from build123d import *

# Parameters (mm, degrees)
F1_R     = 13.2
F2_DEPTH = 7


with BuildPart() as f2:
    # F1 (on Top) → F2 (new body)
    with BuildSketch(Plane.XY):
        with BuildLine():
            ThreePointArc((10.821909, 27.530935), (10.756845, 27.278632), (10.694101, 27.025743))
            ThreePointArc((10.694101, 27.025743), (10.76097, 27.277589), (10.821909, 27.530935))
        make_face()
        with BuildLine():
            ThreePointArc((23.829551, -4.11045), (12.121504, 9.289095), (10.694101, 27.025743))
            ThreePointArc((10.694101, 27.025743), (10.756845, 27.278632), (10.821909, 27.530935))
            ThreePointArc((10.821909, 27.530935), (0, 41.1), (-10.821909, 27.530935))
            ThreePointArc((-10.821909, 27.530935), (-10.756845, 27.278632), (-10.694101, 27.025743))
            ThreePointArc((-10.694101, 27.025743), (-12.121504, 9.289095), (-23.829551, -4.11045))
            ThreePointArc((-23.829551, -4.11045), (-35.415268, -20.848085), (-15.271056, -17.917565))
            ThreePointArc((-15.271056, -17.917565), (0.00942, -15.335501), (15.28268, -17.959904))
            ThreePointArc((15.28268, -17.959904), (35.426816, -20.829414), (23.829551, -4.11045))
        make_face()
        Circle(F1_R, mode=Mode.SUBTRACT)
        with BuildLine():
            ThreePointArc((-10.694101, 27.025743), (-10.756845, 27.278632), (-10.821909, 27.530935))
            ThreePointArc((-10.821909, 27.530935), (-10.76097, 27.277589), (-10.694101, 27.025743))
        make_face()
    extrude(amount=F2_DEPTH)


solid = f2.part
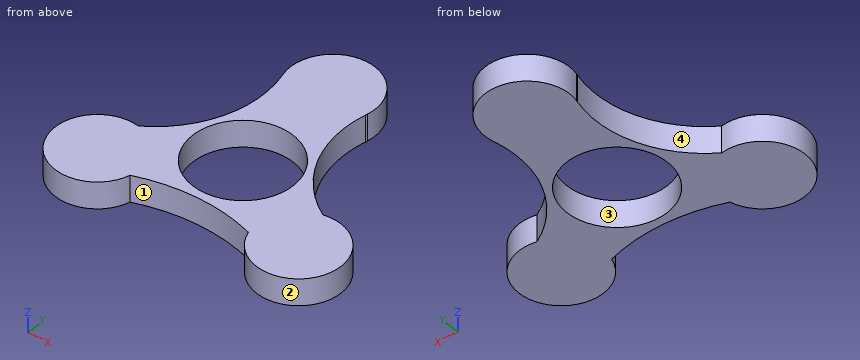
Part model, mm, in its own coordinate system. Face numbers are marked on the shaded views. Coordinates: 2 decimals unless noted, no trailing zeros. Order: outer loops, then holes, each group sorted by start corner. A loop starts at its lowest first (then second) coordinate and runs counter-clockwise, first axis right, second up.
(1) Slice it at B-B, the plane z = 2. Write the cut outline in (x, y), and give its area (3 significant figures).
Check sheet entries:
outline: (-23.83, -4.11) arc R11.1 ccw (long way) to (-15.27, -17.92) arc R46.13 cw to (15.28, -17.96) arc R11.1 ccw (long way) to (23.83, -4.11) arc R28.38 cw to (10.69, 27.03) arc R11.1 ccw to (10.82, 27.53) arc R11.1 ccw (long way) to (-10.82, 27.53) arc R11.1 ccw to (-10.69, 27.03) arc R28.38 cw to start; hole circle Ø26.4 at (0, 0)
area: 1,710 mm2
(2) Probe L1, parallel to X at y = 1.5, z = 1; L2, parallel to Y at x = -6.5, z = 5.25; L3, parallel to X at y = 5.5, z = 4. List the from-to ranges inside material, lowest first.
Check sheet entries:
L1: x = -17.03 to -13.11, 13.11 to 17.03
L2: y = -15.79 to -11.49, 11.49 to 39
L3: x = -14.07 to -12, 12 to 14.07
(3) Slice it at D-D, the plane y = 30. Write the cut outline in (x, z).
Check sheet entries:
outline: (-11.1, 0) - (11.1, 0) - (11.1, 7) - (-11.1, 7) - close
(4) Slice it at C-C, the plane y = 7.5. Write the cut outline in (x, z).
Check sheet entries:
outline: (-12.95, 0) - (-10.86, 0) - (-10.86, 7) - (-12.95, 7) - close; (10.86, 0) - (12.95, 0) - (12.95, 7) - (10.86, 7) - close
(5) Pull direction Y, two halves, no side cores. Call the marked faces 1, 2, 3 and 4: pulls with the +Y half, pulls with the -Y half, needs draft (parallel to the pull), parting line crosses it, or undercut.
Check sheet entries:
face 1: pulls with the -Y half
face 2: parting line crosses it
face 3: undercut
face 4: undercut
(6) Pin check, flat tips, straight feed: pin 1 Ø3 at (x, y) = (3.5, -18.5) entering from +Z; pin 2 Ø1.5 at (x, y) = (10, 23.5) entering from -Z; pin 3 Ø1 at (x, z) = (24, 4) entering from +Y. Stop position of each tip, or through.
Check sheet entries:
pin 1: passes through
pin 2: stops at z = 0
pin 3: stops at y = -3.91
(7) Slice it at A-A, the plane x = -12. Write the cut outline in (y, z), and give its area (3 significant figures).
Check sheet entries:
outline: (-16.91, 0) - (-5.5, 0) - (-5.5, 7) - (-16.91, 7) - close; (5.5, 0) - (9.58, 0) - (9.58, 7) - (5.5, 7) - close
area: 108 mm2
